from build123d import *

# Parameters (mm, degrees)
F1_DEPTH = 3
F2_W     = 20
F2_H     = 3
F3_DEPTH = 7
F4_R     = 5
F5_R     = 5
F6_R     = 1
F7_R     = 1.8
F8_DEPTH = 24


with BuildPart() as f1:
    # F0 (on Top) → F1 (new body)
    with BuildSketch(Plane.XY):
        Polygon((-7.8999784394, 16.9947269248), (-7.8999784394, -6.0052730752), (17.1000215606, -6.0052730752), (17.1000215606, -3.0052730752), (7.1000215606, -3.0052730752), (7.1000215606, 13.9947269248), (17.1000215606, 13.9947269248), (17.1000215606, 16.9947269248), align=None)
    extrude(amount=F1_DEPTH)

    # F2 (on face) → F3 (join)
    with BuildSketch(Plane.XY.offset(3)):
        with Locations((7.1000215606, 15.4947269248)):
            Rectangle(F2_W, F2_H)
        with Locations((7.1000215606, -4.5052730752)):
            Rectangle(F2_W, F2_H)
    extrude(amount=F3_DEPTH)

    # F4
    f4_edges = [f1.edges().sort_by_distance(p)[0] for p in [
        (-7.899978, 16.994727, 1.5),
        (-7.899978, -6.005273, 1.5),
        (-2.899978, -4.505273, 10),
        (-2.899978, 15.494727, 10),
    ]]
    fillet(f4_edges, radius=F4_R)

    # F5
    f5_edges = [f1.edges().sort_by_distance(p)[0] for p in [
        (17.100022, 15.494727, 10),
        (17.100022, -4.505273, 10),
    ]]
    fillet(f5_edges, radius=F5_R)

    # F6
    f6_edges = [f1.edges().sort_by_distance(p)[0] for p in [
        (-6.435512, 15.530261, 3),
        (-7.899978, 5.494727, 3),
        (-6.435512, -4.540807, 3),
    ]]
    fillet(f6_edges, radius=F6_R)

    # F7 (on face) → F8 (cut)
    with BuildSketch(Plane.XZ.offset(6.0052730752)):
        with Locations((12.1000215606, 5)):
            Circle(F7_R)
        with Locations((2.1000215606, 5)):
            Circle(F7_R)
    extrude(amount=-F8_DEPTH, mode=Mode.SUBTRACT)


solid = f1.part
Verification items for the finished model (mm, model axes). A direction names the side the tool comes from. Round coordinates to 2 decimals unless told otherwise and drop trailing zeros. Loops run counter-clockwise (first coordinate to the right, second up) from the corner with the lowest first, then second, coordinate; pieces in that order, holes last. Notation, with made-up numbers: (44.25, -33.5) - (92.25, -33.5) arc R25 cw to (92.25, -20.5) - close; hole circle Ø11 at (16, -30). An arc over 180 degrees is marked (long way). Answer in a Markdown table with one row per item. Add a question column.
Q1. Section check D-D on x = 3.5. Enter the section's corners in (y, z), plus the area to 3 significant figures.
Q2. Release check for a two-part mould opening along X. For faces 3 (the face through (7, 16, 10)), 4 (the face through (10.672, 15.474, 3.905)), 5 (the face through (15.6, 15.52, 8.57)) record: pulls with the +X half, pulls with the -X half, needs draft (parallel to the pull), parting line crosses it, or undercut.
Q3. Tool access check on faces 1 (the face through (-1.4, -4.48, 8.57)), 2 (the face through (9, 13.995, 6)). Record the directions out of +Z, -Z, +X, -X, +Y, -Y that give a thin tool (end or side, any length) a straight path to the whole face; none if there is none.
Q4. Material ranges on line 1 (Y direction, x = -0.5, z = 4.75); line 2 (Z direction, x = 1.5, y = 13.5); line 3 (Z direction, x = 1.25, y = -4.5), recorded low to high.
Q5. Section check A-A on x = 14.25. Enter the section's corners in (y, z), plus the area to 3 significant figures.
Q6. Section check C-C on y = 6.5. Enter the section's corners in (x, z), plus the area to 3 significant figures.
Q7. Gauge pin test, flat ends, axial feed: pin 1 (3.5 mm diameter, centred on y = -4.5, z = 3.5, fed in from -X); pin 2 (2 mm diameter, centred on x = 8.5, y = 0, fed in from +Z); pin 3 (1 mm diameter, centred on x = 4.5, y = 5, fed in from +Z); pin 4 (0.9 mm diameter, centred on y = 15.5, z = 4, fed in from -X). Record the tip position at first contact, or that the pin passes through.
Q8. Section check B-B on z = 8.5. Enter the section's corners in (x, y), plus the area to 3 significant figures.
Found:
| question | item | result |
|---|---|---|
| 1 | outline | (-6.01, 0) - (16.99, 0) - (16.99, 3.87) - (13.99, 3.87) - (13.99, 3) - (-3.01, 3) - (-3.01, 3.87) - (-6.01, 3.87) - close; (-6.01, 6.13) - (-3.01, 6.13) - (-3.01, 10) - (-6.01, 10) - close; (13.99, 6.13) - (16.99, 6.13) - (16.99, 10) - (13.99, 10) - close |
| 1 | area | 97.4 mm² |
| 2 | face 3 | needs draft |
| 2 | face 4 | undercut |
| 2 | face 5 | pulls with the +X half |
| 3 | face 1 | +Z, -X, +Y, -Y |
| 3 | face 2 | +Z, +X |
| 4 | line 1 | y = -6.01 to -3.01, 13.99 to 16.99 |
| 4 | line 2 | z = 0 to 3 |
| 4 | line 3 | z = 0 to 3.41, 6.59 to 9.93 |
| 5 | outline | (-6.01, 0) - (-3.01, 0) - (-3.01, 9.51) - (-6.01, 9.51) - close; (13.99, 0) - (16.99, 0) - (16.99, 9.51) - (13.99, 9.51) - close |
| 5 | area | 57.1 mm² |
| 6 | outline | (-7.9, 0) - (7.1, 0) - (7.1, 3) - (-6.9, 3) arc R1 ccw to (-7.9, 2) - close |
| 6 | area | 44.8 mm² |
| 7 | pin 1 | stops at x = -7.33 |
| 7 | pin 2 | passes through |
| 7 | pin 3 | stops at z = 3 |
| 7 | pin 4 | stops at x = -2.9 |
| 8 | outline | (-1.47, -6.01) - (15.67, -6.01) - (15.67, -3.01) - (-1.47, -3.01) - close; (-1.47, 13.99) - (15.67, 13.99) - (15.67, 16.99) - (-1.47, 16.99) - close |
| 8 | area | 103 mm² |
